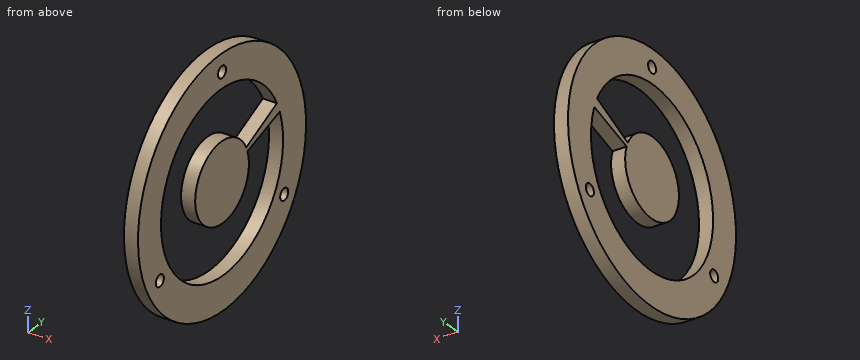
```python
from build123d import *

# Parameters (mm, degrees)
AXIAL_PROFILE_MM_W                                  = 4
AXIAL_PROFILE_MM_H                                  = 34.4
AXIAL_HOLES_DEPTH                                   = 171.775905795
AXIAL_HOLES_DEPTH_BACK                              = 171.775905795
SKETCH2_R                                           = 1.65
C_SHAPED_COOLANT_PASSAGE_AND_INTEGRAL_DI_DEPTH      = 171.775905795
C_SHAPED_COOLANT_PASSAGE_AND_INTEGRAL_DI_DEPTH_BACK = 171.775905795


with BuildPart() as part:
    # Axial profile (mm) → Full revolution (revolve)
    with BuildSketch(Plane.XY, mode=Mode.PRIVATE) as full_revolution_sk:
        with Locations((161.7, 17.2)):
            Rectangle(AXIAL_PROFILE_MM_W, AXIAL_PROFILE_MM_H)
    revolve(full_revolution_sk.sketch.rotate(Axis((-110, 0, 0), (1, 0, 0)), 90), axis=Axis((-110, 0, 0), (1, 0, 0)))

    # Sketch2 → Axial holes (cut, two sides: drawn at the far end of the back side and taken through both)
    with BuildSketch(Plane(origin=(0, 0, 0), x_dir=(0, 0, -1), z_dir=(1, 0, 0)).offset(-AXIAL_HOLES_DEPTH_BACK)):
        with Locations((-29.4, 0)):
            Circle(SKETCH2_R)
        with Locations((14.7, -25.461146871)):
            Circle(SKETCH2_R)
        with Locations((14.7, 25.461146871)):
            Circle(SKETCH2_R)
    extrude(amount=AXIAL_HOLES_DEPTH + AXIAL_HOLES_DEPTH_BACK, mode=Mode.SUBTRACT)

    # Sketch3 → C-shaped coolant passage and integral divider (cut, two sides: drawn at the far end of the back side and taken through both)
    with BuildSketch(Plane(origin=(0, 0, 0), x_dir=(0, 0, -1), z_dir=(1, 0, 0)).offset(-C_SHAPED_COOLANT_PASSAGE_AND_INTEGRAL_DI_DEPTH_BACK)):
        with BuildLine():
            Line((-10.934858177, 22.481745409), (-4.811337598, 9.89196798))
            ThreePointArc((-4.811337598, 9.89196798), (4.209517756, -10.162674858), (-3.592548196, 10.39680708))
            Line((-3.592548196, 10.39680708), (-8.164882263, 23.629107))
            ThreePointArc((-8.164882263, 23.629107), (9.567085809, -23.096988313), (-10.934858177, 22.481745409))
        make_face()
    extrude(amount=C_SHAPED_COOLANT_PASSAGE_AND_INTEGRAL_DI_DEPTH + C_SHAPED_COOLANT_PASSAGE_AND_INTEGRAL_DI_DEPTH_BACK, mode=Mode.SUBTRACT)


solid = part.part
```
Here's how the part is built. I have some questions about the finished solid (model axes, mm). Give positions to 0.01 mm unless a question says otherwise; leave off trailing zeros. Write each loop counter-clockwise with the first axis right and the second up, starting at its lowest first coordinate (ties: lowest second). Pieces come first, ordered by that corner, then holes. Notation, with made-up numbers: (61, -13) -> (113, -13) arc R16 ccw to (113, -6) -> close; hole circle Ø2 at (67, 88). An arc over 180 degrees is marked (long way). Use one line per item in the form item = value.
1) Suppose I cut it at A-A (z = 0). Please give me the cut outline in (x, y), and give its area (3 significant figures).
Verdict:
outline = (159.7, -34.4) -> (163.7, -34.4) -> (163.7, -25) -> (159.7, -25) -> close; (159.7, -11) -> (163.7, -11) -> (163.7, 11) -> (159.7, 11) -> close; (159.7, 25) -> (163.7, 25) -> (163.7, 34.4) -> (159.7, 34.4) -> close
area = 163 mm2
2) Suppose I cut it at C-C (z = -12). Please give me the cut outline in (x, y), and give its area (3 significant figures).
Verdict:
outline = (159.7, -32.24) -> (163.7, -32.24) -> (163.7, -21.93) -> (159.7, -21.93) -> close; (159.7, 21.93) -> (163.7, 21.93) -> (163.7, 32.24) -> (159.7, 32.24) -> close
area = 82.5 mm2
3) Suppose I cut it at B-B (y = 0). Please give me the cut outline in (x, z), and give its area (3 significant figures).
Verdict:
outline = (159.7, -34.4) -> (163.7, -34.4) -> (163.7, -25) -> (159.7, -25) -> close; (159.7, -11) -> (163.7, -11) -> (163.7, 11) -> (159.7, 11) -> close; (159.7, 25) -> (163.7, 25) -> (163.7, 27.75) -> (159.7, 27.75) -> close; (159.7, 31.05) -> (163.7, 31.05) -> (163.7, 34.4) -> (159.7, 34.4) -> close
area = 150 mm2
4) I'm going to push flat-ended pins straight in: pin 1 (1 mm diameter, centred on x = 161, z = 7, fed in from +Y); pin 2 (1.5 mm diameter, centred on x = 161.5, z = -9, fed in from +Y); pin 3 (1 mm diameter, centred on x = 162, z = -20, fed in from -Y); pin 4 (1.5 mm diameter, centred on y = -11.5, z = -5.5, fed in from +X). Where does each tip first touch, or does it pass through?
Verdict:
pin_1 = 33.78
pin_2 = 33.4
pin_3 = -28.34
pin_4 = through
5) Suppose I cut it at D-D (y = -9.5). Please give me the cut outline in (x, z), and give its area (3 significant figures).
Verdict:
outline = (159.7, -33.06) -> (163.7, -33.06) -> (163.7, -23.12) -> (159.7, -23.12) -> close; (159.7, -5.55) -> (163.7, -5.55) -> (163.7, 5.55) -> (159.7, 5.55) -> close; (159.7, 23.12) -> (163.7, 23.12) -> (163.7, 33.06) -> (159.7, 33.06) -> close
area = 124 mm2
6) If I drill on L1, parallel to Y at x = 162.55, z = 0; L2, parallel to Y at x = 160.9, z = -14.7; L3, parallel to Y at x = 161.2, z = -4, over which ranges is the centre line in solid material (lowest first)? Write a range as [from, to].
Verdict:
L1 = [-34.4, -25], [-11, 11], [25, 34.4]
L2 = [-31.1, -27.11], [-23.81, -20.22], [20.22, 23.81], [27.11, 31.1]
L3 = [-34.17, -24.68], [-10.25, 10.25], [24.68, 34.17]
